Can you work these out from the model? Positions are in its coordinate system, mm. Face numbers are marked on the shaded views. Round coordinates to 2 decimals unless told otherwise and drop trailing zeros. Write each loop counter-clockwise with the first axis right and the second up, starting at its lowest first coordinate (ties: lowest second). Pieces come first, ordered by that corner, then holes. Notation, with made-up numbers: M 89.25,42.25 L 135.25,42.25 A28 ccw 135.25,63.25 Z; hole C 10,82.5 d5. An arc over 180 degrees is marked long. Answer in a Markdown table with one row per item. Add a question column.
(1) Suppose I cut it at A-A, the plane x = 0. Write out the boundary of the cut face in (y, z), then the cut area to 3 significant figures.
(2) If I drill on probe 1 along Y at (x, z) = (-30, 2.5); probe 2 along Y at (x, z) = (0, 8.25); probe 3 along X at (y, z) = (1, 1.5), over which ranges is the centre line in solid material (lowest first)?
(3) If we mould it in two halves opening along X, with no side actions, what happens to the marked faces 1, 2 and 3? For each: released by +X, released by -X, zero draft, split by the parting line, or undercut.
(4) Suppose I cut it at C-C, the plane z = 4.75. Write out the boundary of the cut face in (x, y), then the cut area to 3 significant figures.
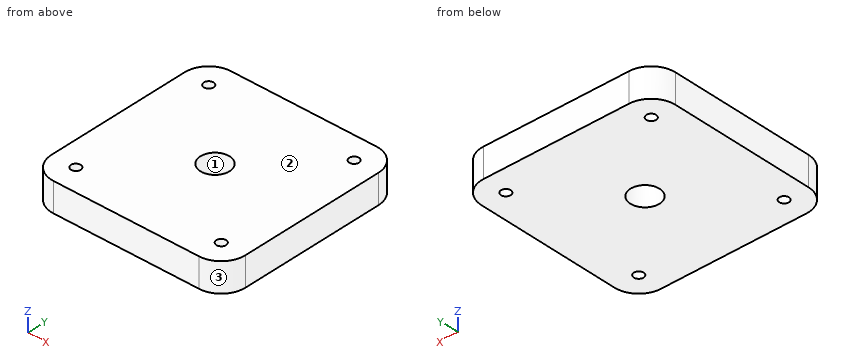
Autodesk Inventor part; units mm, degrees
ref_plane "Plano de trabalho1" through (0, 0, 0) normal (0, 0, 1) x (1, 0, 0)
ref_plane "YZ Plane" through (0, 0, 0) normal (1, 0, 0) x (0, 1, 0)
ref_plane "XZ Plane" through (0, 0, 0) normal (0, 1, 0) x (-1, 0, 0)
ref_plane "Plano de trabalho1" through (0, 0, 0) normal (0, 0, 1) x (1, 0, 0)
sketch "Esboço1" plane through (0, 0, 0) normal (0, 0, 1) x (1, 0, 0)
  arc A0 (-40, -30) -> (-30, -40) centre (-30, -30) ccw
  line L0 (30, -40) -> (-30, -40)
  arc A1 (30, -40) -> (40, -30) centre (30, -30) ccw
  line L1 (40, 30) -> (40, -30)
  arc A2 (40, 30) -> (30, 40) centre (30, 30) ccw
  line L2 (-30, 40) -> (30, 40)
  arc A3 (-30, 40) -> (-40, 30) centre (-30, 30) ccw
  line L3 (-40, -30) -> (-40, 30)
  circle A4 centre (0, 0) radius 5
  circle A5 centre (0, 0) radius 6
  circle A6 centre (30, 30) radius 2
  circle A7 centre (30, -30) radius 2
  circle A8 centre (-30, -30) radius 2
  circle A9 centre (-30, 30) radius 2
  point P0 (0, 0)
  dimension "d0" = 12
  dimension "d3" = 4
  dimension "d4" = 4
  dimension "d5" = 4
  dimension "d6" = 4
  dimension "d7" = 80
extrude "Extrusão1" add sketch "Esboço1" along normal blind 12 contours L3 A3 L2 A2 L1 A1 L0 A0
equation "\"d3\" = d6"
equation "\"d4\" = d6"
equation "\"d5\" = d6"
properties part number "corpo_01b"
Calculated:
| question | item | result |
|---|---|---|
| 1 | outline | M -40,0 L -6,0 L -6,12 L -40,12 Z; M 6,0 L 40,0 L 40,12 L 6,12 Z |
| 1 | area | 816 mm² |
| 2 | probe 1 | -40 to -32, -28 to 28, 32 to 40 |
| 2 | probe 2 | -40 to -6, 6 to 40 |
| 2 | probe 3 | -40 to -5.92, 5.92 to 40 |
| 3 | face 1 | undercut |
| 3 | face 2 | zero draft |
| 3 | face 3 | released by +X |
| 4 | outline | M -40,-30 A10 ccw -30,-40 L 30,-40 A10 ccw 40,-30 L 40,30 A10 ccw 30,40 L -30,40 A10 ccw -40,30 Z; hole C -30,-30 d4; hole C -30,30 d4; hole C 0,0 d12; hole C 30,-30 d4; hole C 30,30 d4 |
| 4 | area | 6,150 mm² |
